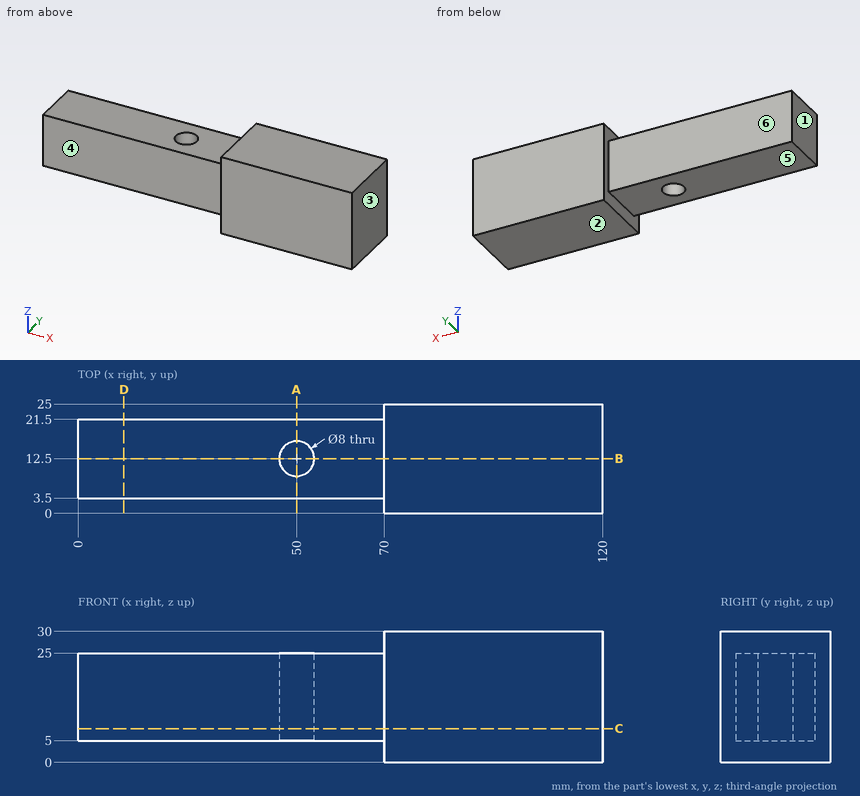
For this review, use the dimensioned drawing (mm, ordinates from the lowest corner) and the shaded views. A direction names the side the tool comes from. Give positions to 0.01 mm unless a question says otherwise; leave off trailing zeros. Order: outer loops, then holes, each group sorted by start corner. A loop starts at its lowest first (then second) coordinate and runs counter-clockwise, first axis right, second up. Notation, with made-up numbers: (-7, 12.25) - (-1, 12.25) arc R28 cw to (-1, 40.25) - close; hole circle Ø11 at (-36.75, -29.5). An arc over 180 degrees is marked (long way). Use a Markdown table: item, result. Add a question column.
(1) Wall thickness on probe 1 along Y at (x, z) = (50, 9.5); probe 2 along X at (y, z) = (22, 3); probe 3 along Y at (x, z) = (40, 9.5): over which ranges is each line inside the solid? List them lowest first. Write a range as [from, to].
(2) Clearance check with flat-ended pins moving along their axes: P1, Ø6, axis at x = 49.5, z = 14.5, coming from the -Y side; P2, Ø6, axis at x = 45.5, z = 11, coming from the +Y side; P3, Ø5.5, axis at x = 23, y = 13.5, coming from the -Z side. State where each tip first meets the part, or that it passes through.
(3) Add section D-D on x = 10.5. Give the boundary of the cut face in (y, z), then the cut area to 3 significant figures.
(4) Add section B-B on y = 12.5. Give the boundary of the cut face in (x, z).
(5) Mouldability with a two-part tool opening along X and no side actions: class the marked faces 1, 2 and 3 as +X half, -X half, draft (parallel to the pull), parting line (faces both ways), or undercut.
(6) Machinability: for the marked faces 4, 5 and 6, which of the approach directions +Z, -Z, +X, -X, +Y, -Y give a long, thin tool a straight path to every point of the face, cutting with its end or side? Answer none if there is none.
(7) Add section A-A on x = 50. Give the boundary of the cut face in (y, z), then the cut area to 3 significant figures.
(8) Add section C-C on z = 7.75. Give the boundary of the cut face in (x, y).
Report:
| question | item | result |
|---|---|---|
| 1 | probe 1 | y = [3.5, 8.5], [16.5, 21.5] |
| 1 | probe 2 | x = [70, 120] |
| 1 | probe 3 | y = [3.5, 21.5] |
| 2 | P1 | stops at y = 3.5 |
| 2 | P2 | stops at y = 21.5 |
| 2 | P3 | stops at z = 5 |
| 3 | outline | (3.5, 5) - (21.5, 5) - (21.5, 25) - (3.5, 25) - close |
| 3 | area | 360 mm² |
| 4 | outline | (0, 5) - (46, 5) - (46, 25) - (0, 25) - close; (54, 5) - (70, 5) - (70, 0) - (120, 0) - (120, 30) - (70, 30) - (70, 25) - (54, 25) - close |
| 5 | face 1 | -X half |
| 5 | face 2 | draft |
| 5 | face 3 | +X half |
| 6 | face 4 | +Z, -Z, -X, -Y |
| 6 | face 5 | -Z, -X, +Y, -Y |
| 6 | face 6 | +Z, -Z, -X, +Y |
| 7 | outline | (3.5, 5) - (8.5, 5) - (8.5, 25) - (3.5, 25) - close; (16.5, 5) - (21.5, 5) - (21.5, 25) - (16.5, 25) - close |
| 7 | area | 200 mm² |
| 8 | outline | (0, 3.5) - (70, 3.5) - (70, 0) - (120, 0) - (120, 25) - (70, 25) - (70, 21.5) - (0, 21.5) - close; hole circle Ø8 at (50, 12.5) |
